Here's the drawing with two shaded views (mm, measured from the low corner). I have some questions. Round coordinates to 2 decimals unless told otherwise and drop trailing zeros. Loops run counter-clockwise (first coordinate to the right, second up) from the corner with the lowest first, then second, coordinate; pieces in that order, holes last.
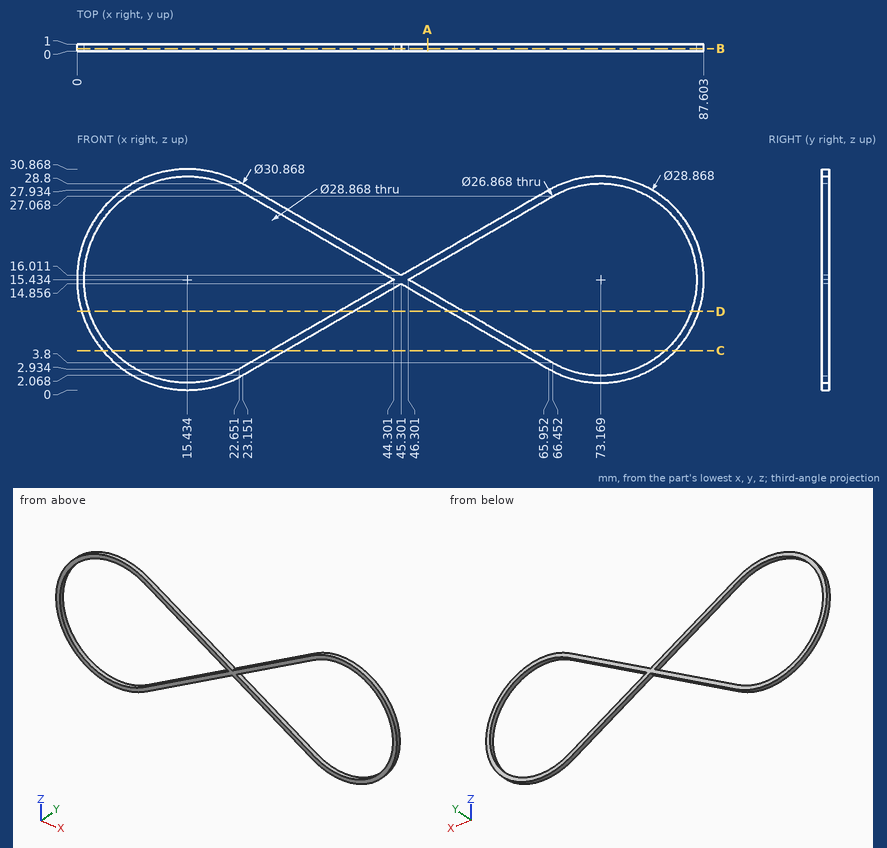
(1) If we section it at B-B, the plane y = 0.35: List the corners of the cut face in (x, z) for me.
Worked answers:
outline: (23.15, 2.07) - (45.3, 14.86) - (65.95, 2.93) arc R14.43 ccw (long way) to (65.95, 27.93) - (45.3, 16.01) - (23.15, 28.8) arc R15.43 ccw (long way) to start; hole (22.65, 2.93) - (44.3, 15.43) - (22.65, 27.93) arc R14.43 ccw (long way) to start; hole (46.3, 15.43) - (66.45, 3.8) arc R13.43 ccw (long way) to (66.45, 27.07) - close
(2) If I drill on line 1 (X direction, y = 0.85, z = 14.5) (1 decimal); line 2 (X direction, y = 0.75, z = 23.5) (1 decimal); line 3 (Z direction, x = 10, y = 0.2) (1 decimal), over which ranges is the centre line in solid material (lowest first)?
Worked answers:
line 1: x = 0 to 1, 42.7 to 44.7, 45.9 to 47.9, 86.6 to 87.6
line 2: x = 2.3 to 3.5, 30.3 to 32.3, 58.3 to 60.3, 83.9 to 85.1
line 3: z = 1 to 2.1, 28.8 to 29.9
(3) If we section it at D-D, the plane z = 11: State how many separate pieces and enclosed holes the cut face has.
Worked answers:
separate pieces: 4
enclosed holes: 0
(4) If we section it at C-C, the plane z = 5.5: List the corners of the cut face in (x, y) for me (1 decimal).
Worked answers:
outline: (3.6, 0) - (5, 0) - (5, 1) - (3.6, 1) - close; (27.1, 0) - (29.1, 0) - (29.1, 1) - (27.1, 1) - close; (61.5, 0) - (63.5, 0) - (63.5, 1) - (61.5, 1) - close; (82.2, 0) - (83.6, 0) - (83.6, 1) - (82.2, 1) - close
(5) If we section it at A-A, the plane x = 49: List the corners of the cut face in (y, z) for me (1 decimal).
Worked answers:
outline: (0, 12.7) - (1, 12.7) - (1, 13.9) - (0, 13.9) - close; (0, 17) - (1, 17) - (1, 18.1) - (0, 18.1) - close
